Here's the drawing with two shaded views (mm, measured from the low corner). I have some questions. Round coordinates to 2 decimals unless told otherwise and drop trailing zeros. Order: outer loops, then holes, each group sorted by start corner. A loop starts at its lowest first (then second) coordinate and runs counter-clockwise, first axis right, second up. Notation, with made-up numbers: M -9,-19 L 9,-19 A24 cw 9,-7 Z; hole C 21.5,-4 d8. An arc over 180 degrees is marked long. One line per question, with ' | ' between items.
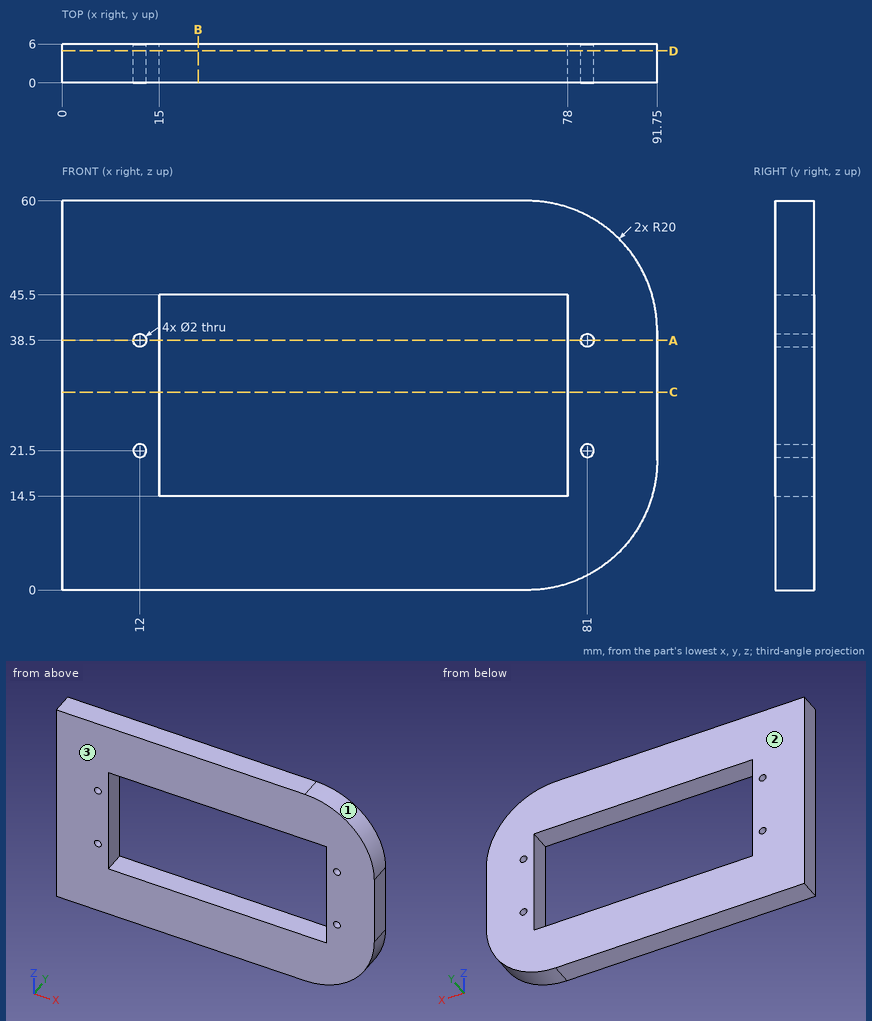
(1) If we section it at A-A on z = 38.5: Please give me the cut outline in (x, y).
Final values:
outline: M 0,0 L 11,0 L 11,6 L 0,6 Z; M 13,0 L 15,0 L 15,6 L 13,6 Z; M 78,0 L 80,0 L 80,6 L 78,6 Z; M 82,0 L 91.75,0 L 91.75,6 L 82,6 Z
(2) Thinking about a two-plate mould opening in Y: for the marked faces 1, 2 and 3, which applies, released by +Y, released by -Y, zero draft, split by the parting line, or undercut?
Final values:
face 1: zero draft | face 2: released by +Y | face 3: released by -Y
(3) Please list where these lines run through material, in increasing order: probe 1 along X at (y, z) = (4.6, 38.5); probe 2 along Z at (x, y) = (12, 2.05); probe 3 along X at (y, z) = (0.9, 24.5). Write a range as [from, to].
Final values:
probe 1: [0, 11], [13, 15], [78, 80], [82, 91.75] | probe 2: [0, 20.5], [22.5, 37.5], [39.5, 60] | probe 3: [0, 15], [78, 91.75]
(4) If we section it at C-C on z = 30.5: Please give me the cut outline in (x, y).
Final values:
outline: M 0,0 L 15,0 L 15,6 L 0,6 Z; M 78,0 L 91.75,0 L 91.75,6 L 78,6 Z
(5) If we section it at D-D on y = 4.95: Please give me the cut outline in (x, z).
Final values:
outline: M 0,0 L 71.75,0 A20 ccw 91.75,20 L 91.75,40 A20 ccw 71.75,60 L 0,60 Z; hole C 12,21.5 d2; hole C 12,38.5 d2; hole M 15,14.5 L 78,14.5 L 78,45.5 L 15,45.5 Z; hole C 81,21.5 d2; hole C 81,38.5 d2
(6) If we section it at B-B on x = 21: Please give me the cut outline in (y, z), plus the area to 3 significant figures.
Final values:
outline: M 0,0 L 6,0 L 6,14.5 L 0,14.5 Z; M 0,45.5 L 6,45.5 L 6,60 L 0,60 Z | area: 174 mm^2
(7) Will these pins go through, and if not, where does the flat tip stop? pin 1 Ø1.5 at (x, y) = (82, 2) entering from -Z; pin 2 Ø3 at (x, y) = (34.5, 3.5) entering from -Z; pin 3 Ø1.2 at (x, z) = (81, 21.5) entering from +Y.
Final values:
pin 1: z = 2.4 | pin 2: z = 0 | pin 3: through
